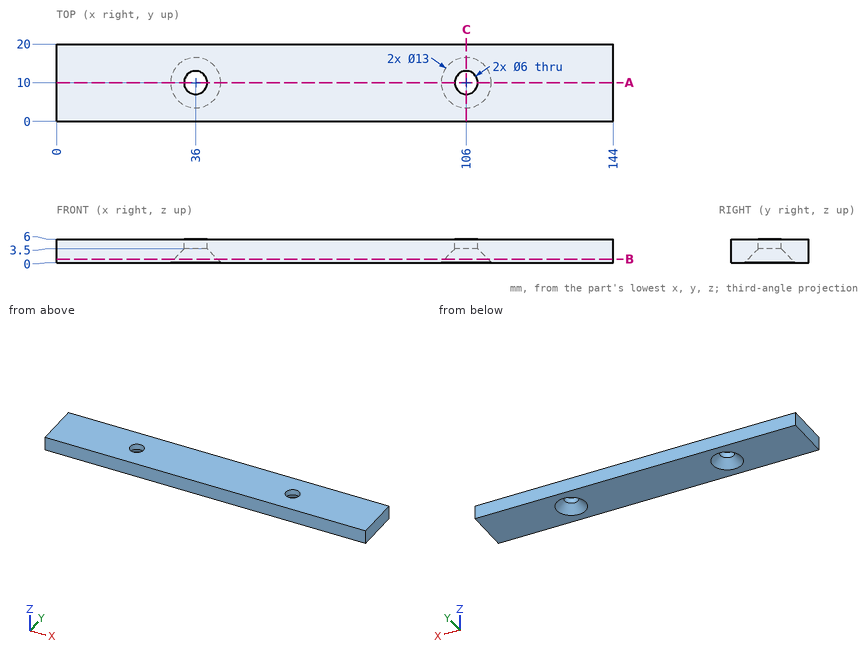
Verification items for this drawing (mm, ordinates from the low corner). Coordinates: 2 decimals unless noted, no trailing zeros. Loops run counter-clockwise (first coordinate to the right, second up) from the corner with the lowest first, then second, coordinate; pieces in that order, holes last. Notation, with made-up numbers: (4, 16) - (63, 16) arc R12 cw to (63, 30) - close; hole circle Ø3 at (71, 8.25). An arc over 180 degrees is marked (long way). Answer as a JSON object with one key per item and string values.
(1) Go/stop test with flat-tipped pins: pin 1 Ø8 at (x, y) = (36, 10) entering from +Z; pin 2 Ø5 at (x, y) = (106, 10) entering from -Z. Record where each tip stops, or that it passes through.
Response:
{"pin 1": "stops at z = 6", "pin 2": "passes through"}
(2) Cross-section at A-A, the plane y = 10. Record the boundary of the cut face in (x, z).
Response:
{"outline": "(0, 0) - (29.5, 0) - (33, 3.5) - (33, 6) - (0, 6) - close; (39, 3.5) - (42.5, 0) - (99.5, 0) - (103, 3.5) - (103, 6) - (39, 6) - close; (109, 3.5) - (112.5, 0) - (144, 0) - (144, 6) - (109, 6) - close"}
(3) Cross-section at C-C, the plane x = 106. Record the boundary of the cut face in (y, z).
Response:
{"outline": "(0, 0) - (3.5, 0) - (7, 3.5) - (7, 6) - (0, 6) - close; (13, 3.5) - (16.5, 0) - (20, 0) - (20, 6) - (13, 6) - close"}
(4) Cross-section at B-B, the plane z = 0.9. Record the boundary of the cut face in (x, y).
Response:
{"outline": "(0, 0) - (144, 0) - (144, 20) - (0, 20) - close; hole circle Ø11.2 at (36, 10); hole circle Ø11.2 at (106, 10)"}
(5) Scan lines: line 1 along X through (y, z) = (10, 4.2); line 2 along Y through (x, z) = (106, 5); line 3 along X through (y, z) = (7.5, 1.05). Record each from-to range of solid material in increasing order.
Response:
{"line 1": "x = 0 to 33, 39 to 103, 109 to 144", "line 2": "y = 0 to 7, 13 to 20", "line 3": "x = 0 to 31.16, 40.84 to 101.16, 110.84 to 144"}
